Read the model definition and answer for the solid it produces. Units are mm, in the model's axes. A direction names the side the tool comes from. Give positions to 0.01 mm unless a question says otherwise; leave off trailing zeros. Order: outer loops, then holes, each group sorted by start corner. A loop starts at its lowest first (then second) coordinate and runs counter-clockwise, first axis right, second up. Notation, with made-up numbers: (-38.5, -9) - (6.5, -9) arc R14 cw to (6.5, 7) - close; hole circle Ø6 at (31, 67). An arc over 180 degrees is marked (long way). Answer as CSV lines item,"result". Start each with the question number.
Autodesk Inventor part; units mm, degrees
ref_plane "YZ Plane" through (0, 0, 0) normal (1, 0, 0) x (0, 1, 0)
ref_plane "XZ Plane" through (0, 0, 0) normal (0, 1, 0) x (-1, 0, 0)
ref_plane "XY Plane" through (0, 0, 0) normal (0, 0, 1) x (1, 0, 0)
sketch "Sketch1" plane through (0, 0, 0) normal (0, 0, 1) x (1, 0, 0)
  line L0 (-10.3132, 5.9874) -> (10.3132, 5.9874)
  line L1 (10.3132, 5.9874) -> (10.3132, -6.7322)
  line L2 (10.3132, -6.7322) -> (-10.3132, -6.7322)
  line L3 (-10.3132, -6.7322) -> (-10.3132, 5.9874)
  line L4 (-10.3132, 5.9874) -> (10.3132, -6.7322) construction
  line L5 (10.3132, 5.9874) -> (-10.3132, -6.7322) construction
  point P0 (0, 0)
  point P1 (0, -0.3724)
extrude "Extrusion1" add sketch "Sketch1" along normal blind 5
sketch "Sketch2" plane through (0, 0, 5) normal (0, 0, 1) x (1, 0, 0)
  line L0 (10.3132, 5.9874) -> (-10.3132, 5.9874)
  line L1 (-10.3132, -6.7322) -> (10.3132, -6.7322)
  line L2 (0, 5.9874) -> (2, 5.9874)
  line L3 (2, 5.9874) -> (2, -6.7322)
  line L4 (2, -6.7322) -> (-2, -6.7322)
  line L5 (-2, -6.7322) -> (-2, 5.9874)
  line L6 (0, 5.9874) -> (-2, 5.9874)
  dimension "d2" = 2
  dimension "d3" = 4
extrude "Extrusion2" add sketch "Sketch2" along normal blind 15
(1) Which of the six approach directions +Z, -Z, +X, -X, +Y, -Y give full straight-line access (tool end or side, diameter ignored) to faces 1 (the flat face through (10.313, 0, 2)), 2 (the flat face through (2, 0, 12)), 3 (the flat face through (-2, 0, 12))?
(2) Section C-C, the plane x = -6 is taken. Write down the section's boundary in (y, z).
(3) Straight lines are drawn through the part: line 1 (Z direction, x = -7, y = 1); line 2 (X direction, y = 2.25, z = 15.75). For each, find the intervals that lie inside material, in ascending order. Write a range as [from, to].
(4) Section A-A, the plane y = 3.75 is taken. Write down the section's boundary in (x, z), and give its area (3 significant figures).
(5) A flat-ended cylindrical pin translates along its axis: pin 1 Ø3 at (x, y) = (-4.5, -2) entering from +Z. Find the tip coordinate at first contact, or state that the pin passes through.
(6) Section B-B, the plane z = 8.75 is taken. Write down the section's boundary in (x, y).
Checks:
1,face 1,"+Z, -Z, +X, +Y, -Y"
1,face 2,"+Z, +X, +Y, -Y"
1,face 3,"+Z, -X, +Y, -Y"
2,outline,"(-6.73, 0) - (5.99, 0) - (5.99, 5) - (-6.73, 5) - close"
3,line 1,"z = [0, 5]"
3,line 2,"x = [-2, 2]"
4,outline,"(-10.31, 0) - (10.31, 0) - (10.31, 5) - (2, 5) - (2, 20) - (-2, 20) - (-2, 5) - (-10.31, 5) - close"
4,area,"163 mm²"
5,pin 1,"stops at z = 5"
6,outline,"(-2, -6.73) - (2, -6.73) - (2, 5.99) - (-2, 5.99) - close"
